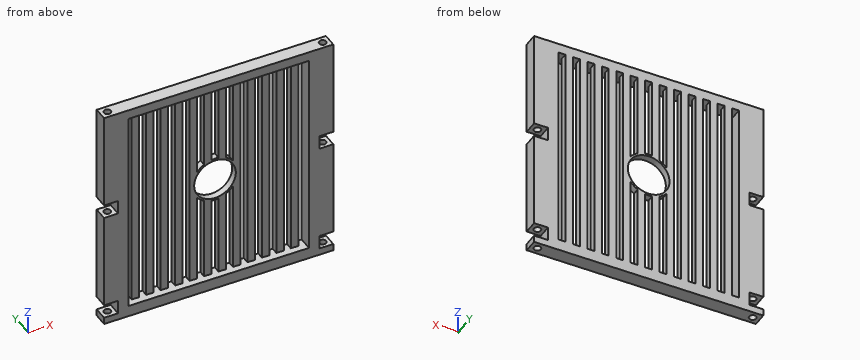
from build123d import *

# Parameters (mm, degrees)
ESQUISSE1_W             = 5
ESQUISSE1_H             = 150
ESQUISSE1_R             = 15
BASE_DEPTH              = 10
VIDE_VIS_DEPTH          = 127.219055614
VIDE_VIS_DEPTH_BACK     = 127.219055614
ESQUISSE5_R             = 2.5
ESQUISSE6_W             = 130
ESQUISSE6_H             = 150
ENL_V_MAT_EXTRU_6_DEPTH = 5


with BuildPart() as part:
    # Esquisse1 → BASE (new body)
    with BuildSketch(Plane(origin=(0, 0, 0), x_dir=(1, 0, 0), z_dir=(0, 1, 0))):
        Polygon((-82.5, 82.5), (-82.5, 77.5), (-72.5, 77.5), (-72.5, 67.5), (-82.5, 67.5), (-82.5, -2.5), (-72.5, -2.5), (-72.5, -12.5), (-82.5, -12.5), (-82.5, -82.5), (82.5, -82.5), (82.5, -12.5), (72.5, -12.5), (72.5, -2.5), (82.5, -2.5), (82.5, 67.5), (72.5, 67.5), (72.5, 77.5), (82.5, 77.5), (82.5, 82.5), align=None)
        with BuildLine():
            ThreePointArc((-12.916666667, -10.915030923), (-10.627210874, -13.27000839), (-7.916666667, -15.124860621))
            Line((-7.916666667, -15.124860621), (-7.916666667, -75.648107225))
            Line((-7.916666667, -75.648107225), (-12.916666667, -75.648107225))
            Line((-12.916666667, -75.648107225), (-12.916666667, -10.915030923))
        make_face(mode=Mode.SUBTRACT)
        with Locations((-62.5, -0.648107225)):
            Rectangle(ESQUISSE1_W, ESQUISSE1_H, mode=Mode.SUBTRACT)
        with Locations((-52.083333333, -0.648107225)):
            Rectangle(ESQUISSE1_W, ESQUISSE1_H, mode=Mode.SUBTRACT)
        with Locations((-41.666666667, -0.648107225)):
            Rectangle(ESQUISSE1_W, ESQUISSE1_H, mode=Mode.SUBTRACT)
        with Locations((-31.25, -0.648107225)):
            Rectangle(ESQUISSE1_W, ESQUISSE1_H, mode=Mode.SUBTRACT)
        with Locations((-20.833333333, -0.648107225)):
            Rectangle(ESQUISSE1_W, ESQUISSE1_H, mode=Mode.SUBTRACT)
        with Locations(Location((0, -0.648107225, 0), (0, 0, 270))):
            Circle(ESQUISSE1_R, mode=Mode.SUBTRACT)
        with BuildLine():
            Line((-2.5, -75.648107225), (-2.5, -16.957613655))
            ThreePointArc((-2.5, -16.957613655), (0, -17.148107225), (2.5, -16.957613655))
            Line((2.5, -16.957613655), (2.5, -75.648107225))
            Line((2.5, -75.648107225), (-2.5, -75.648107225))
        make_face(mode=Mode.SUBTRACT)
        with BuildLine():
            Line((7.916666667, -75.648107225), (7.916666667, -15.124860621))
            ThreePointArc((7.916666667, -15.124860621), (10.627210874, -13.27000839), (12.916666667, -10.915030923))
            Line((12.916666667, -10.915030923), (12.916666667, -75.648107225))
            Line((12.916666667, -75.648107225), (7.916666667, -75.648107225))
        make_face(mode=Mode.SUBTRACT)
        with BuildLine():
            Line((-12.916666667, 9.618816473), (-12.916666667, 74.351892775))
            Line((-12.916666667, 74.351892775), (-7.916666667, 74.351892775))
            Line((-7.916666667, 74.351892775), (-7.916666667, 13.828646171))
            ThreePointArc((-7.916666667, 13.828646171), (-10.627210874, 11.973793941), (-12.916666667, 9.618816473))
        make_face(mode=Mode.SUBTRACT)
        with Locations((20.833333333, -0.648107225)):
            Rectangle(ESQUISSE1_W, ESQUISSE1_H, mode=Mode.SUBTRACT)
        with Locations((31.25, -0.648107225)):
            Rectangle(ESQUISSE1_W, ESQUISSE1_H, mode=Mode.SUBTRACT)
        with Locations((41.666666667, -0.648107225)):
            Rectangle(ESQUISSE1_W, ESQUISSE1_H, mode=Mode.SUBTRACT)
        with Locations((52.083333333, -0.648107225)):
            Rectangle(ESQUISSE1_W, ESQUISSE1_H, mode=Mode.SUBTRACT)
        with Locations((62.5, -0.648107225)):
            Rectangle(ESQUISSE1_W, ESQUISSE1_H, mode=Mode.SUBTRACT)
        with BuildLine():
            Line((-2.5, 15.661399205), (-2.5, 74.351892775))
            Line((-2.5, 74.351892775), (2.5, 74.351892775))
            Line((2.5, 74.351892775), (2.5, 15.661399205))
            ThreePointArc((2.5, 15.661399205), (0, 15.851892775), (-2.5, 15.661399205))
        make_face(mode=Mode.SUBTRACT)
        with BuildLine():
            Line((12.916666667, 74.351892775), (12.916666667, 9.618816473))
            ThreePointArc((12.916666667, 9.618816473), (10.627210874, 11.973793941), (7.916666667, 13.828646171))
            Line((7.916666667, 13.828646171), (7.916666667, 74.351892775))
            Line((7.916666667, 74.351892775), (12.916666667, 74.351892775))
        make_face(mode=Mode.SUBTRACT)
    extrude(amount=BASE_DEPTH)

    # Esquisse5 → VIDE VIS (cut, two sides: drawn at the far end of the back side and taken through both)
    with BuildSketch(Plane(origin=(0, 0, 12.5), x_dir=(-1, 0, 0), z_dir=(0, 0, -1)).offset(-VIDE_VIS_DEPTH_BACK)):
        with Locations((-77.5, 5)):
            Circle(ESQUISSE5_R)
        with Locations(Location((77.5, 5, 0), (0, 0, 180))):
            Circle(ESQUISSE5_R)
    extrude(amount=VIDE_VIS_DEPTH + VIDE_VIS_DEPTH_BACK, mode=Mode.SUBTRACT)

    # Esquisse6 → Enlèv. mat.-Extru.6 (cut)
    with BuildSketch(Plane.XZ):
        with Locations((0, 0.648107225)):
            Rectangle(ESQUISSE6_W, ESQUISSE6_H)
    extrude(amount=-ENL_V_MAT_EXTRU_6_DEPTH, mode=Mode.SUBTRACT)


solid = part.part
Build history of the part. All positions in model axes, mm. Round coordinates to 2 decimals unless told otherwise and drop trailing zeros. Write each loop counter-clockwise with the first axis right and the second up, starting at its lowest first coordinate (ties: lowest second). Pieces come first, ordered by that corner, then holes. Notation, with made-up numbers: M 26,21.25 L 60,21.25 A23 ccw 60,54.25 Z; hole C 32,75.5 d2. An arc over 180 degrees is marked long. Answer as a JSON object with one key per item and string values. Group by question number.
(1) Flat gauge pin, fed straight in: pin 1 (2.5 mm diameter, centred on x = -58.5, z = 35.5, fed in from -Y). Where does the tip first touch, or does it go through?
(2) Cut at C-C (z = -51). Give the number of separate pieces and of enclosed holes in the cut face, and give its area (3 significant figures).
(3) Drill centre lines: L1, parallel to Z at x = 51.5, y = 7.5; L2, parallel to X at y = 3, z = 42; L3, parallel to Y at x = -77.5, z = -48.5. Where is each one in solid material? Low to high.
(4) Cut at A-A (x = 77.5). Give the cut face in (y, z), and give its area (3 significant figures).
(5) Cut at B-B (x = 0). Give the cut face in (y, z), and give its area (3 significant figures).
Responses:
{
 "1": {"pin 1": "stops at y = 5"},
 "2": {"separate pieces": "14", "enclosed holes": "2", "area": "636 mm2"},
 "3": {"L1": "z = -82.5 to -74.35, 75.65 to 82.5", "L2": "x = -82.5 to -79, -76 to -65, 65 to 76, 79 to 82.5", "L3": "y = 0 to 2.5, 7.5 to 10"},
 "4": {"outline": "M 0,-82.5 L 2.5,-82.5 L 2.5,-77.5 L 0,-77.5 Z; M 0,-67.5 L 2.5,-67.5 L 2.5,2.5 L 0,2.5 Z; M 0,12.5 L 2.5,12.5 L 2.5,82.5 L 0,82.5 Z; M 7.5,-82.5 L 10,-82.5 L 10,-77.5 L 7.5,-77.5 Z; M 7.5,-67.5 L 10,-67.5 L 10,2.5 L 7.5,2.5 Z; M 7.5,12.5 L 10,12.5 L 10,82.5 L 7.5,82.5 Z", "area": "725 mm2"},
 "5": {"outline": "M 0,-82.5 L 10,-82.5 L 10,-74.35 L 0,-74.35 Z; M 0,75.65 L 10,75.65 L 10,82.5 L 0,82.5 Z; M 5,-15.85 L 10,-15.85 L 10,-14.35 L 5,-14.35 Z; M 5,15.65 L 10,15.65 L 10,17.15 L 5,17.15 Z", "area": "165 mm2"}
}
